```python
from build123d import *

# Parameters (mm, degrees)
F0_W     = 30
F0_H     = 40
F1_DEPTH = 17
F3_DEPTH = 15
F4_W     = 16.507677
F4_H     = 19.664884
F5_DEPTH = 10


with BuildPart() as f1:
    # F0 (on Top) → F1 (new body)
    with BuildSketch(Plane.XY):
        with Locations((15, 20)):
            Rectangle(F0_W, F0_H)
    extrude(amount=F1_DEPTH)

    # F2 (on face) → F3 (cut)
    with BuildSketch(Plane.XY.offset(17)):
        with BuildLine():
            Line((13, 27.113265), (13, 22.613265))
            ThreePointArc((13, 22.613265), (15, 15.149164), (17, 22.613265))
            Line((17, 22.613265), (17, 27.113265))
            ThreePointArc((17, 27.113265), (15, 29.113265), (13, 27.113265))
        make_face()
    extrude(amount=-F3_DEPTH, mode=Mode.SUBTRACT)

    # F4 (on face) → F5 (cut)
    with BuildSketch(Plane.XY.offset(2)):
        with Locations((15.471233, 21.540843)):
            Rectangle(F4_W, F4_H)
    extrude(amount=F5_DEPTH, mode=Mode.SUBTRACT)


solid = f1.part
```
Could you check a few things on this model? Use its own coordinates, in mm. A direction names the side the tool comes from. Give positions to 0.01 mm unless a question says otherwise; leave off trailing zeros. Order: outer loops, then holes, each group sorted by start corner. A loop starts at its lowest first (then second) coordinate and runs counter-clockwise, first axis right, second up.
Q1. If I drill on line 1 along Y through (x, z) = (17.75, 6.5); line 2 along X through (y, z) = (22, 9.25); line 3 along Y through (x, z) = (15, 14.9), over which ranges is the centre line in solid material (lowest first)?
Q2. Suppose I cut it at B-B, the plane z = 12.75. Write out the boundary of the cut face in (x, y), and give its area (3 significant figures).
Q3. Suppose I cut it at C-C, the plane z = 5.25. Write out the boundary of the cut face in (x, y).
Q4. For faces 1 (the flat face through (15, 31.373, 7)), 2 (the flat face through (11, 25, 17)), 3 (the flat face through (17, 25, 15)), which set-ups out of +Z, -Z, +X, -X, +Y, -Y let a thin tool reach every point of the face, with its end or its side?
Q5. Suppose I cut it at A-A, the plane x = 15. Write out the boundary of the cut face in (y, z).
Q6. We'd pull the mould along Y, two halves only. Please class faces 4 (the flat face through (15, 11.708, 7)), 5 (the flat face through (15, 20, 0)), 6 (the flat face through (15, 0, 8)): +Y half, -Y half, draft (parallel to the pull), parting line (faces both ways), or undercut.
Solution:
1. line 1: y = 0 to 11.71, 31.37 to 40
1. line 2: x = 0 to 7.22, 23.73 to 30
1. line 3: y = 0 to 15.15, 29.11 to 40
2. outline: (0, 0) - (30, 0) - (30, 40) - (0, 40) - close; hole (13, 22.61) arc R4 ccw (long way) to (17, 22.61) - (17, 27.11) arc R2 ccw to (13, 27.11) - close
2. area: 1,130 mm2
3. outline: (0, 0) - (30, 0) - (30, 40) - (0, 40) - close; hole (7.22, 11.71) - (23.73, 11.71) - (23.73, 31.37) - (7.22, 31.37) - close
4. face 1: none
4. face 2: +Z, +X, -X, +Y, -Y
4. face 3: +Z
5. outline: (0, 0) - (40, 0) - (40, 17) - (29.11, 17) - (29.11, 12) - (31.37, 12) - (31.37, 2) - (11.71, 2) - (11.71, 12) - (15.15, 12) - (15.15, 17) - (0, 17) - close
6. face 4: undercut
6. face 5: draft
6. face 6: -Y half
